```python
from build123d import *

# Parameters (mm, degrees)
SKETCH1_R          = 73.025
SKETCH1_R_2        = 42.8625
EXTRUDE1_DEPTH     = 38.1
SKETCH2_R          = 65.0875
CUT_EXTRUDE1_DEPTH = 30.1625
SKETCH3_R          = 5.55625
CUT_EXTRUDE2_DEPTH = 30.1625
CIRPATTERN1_COUNT  = 8
SKETCH5_R          = 5.55625
EXTRUDE2_DEPTH     = 7.9375
CIRPATTERN2_COUNT  = 4


with BuildPart() as part:
    # Sketch1 → Extrude1 (new body)
    with BuildSketch(Plane(origin=(0, 0, 0), x_dir=(1, 0, 0), z_dir=(0, 1, 0))):
        Circle(SKETCH1_R)
        Circle(SKETCH1_R_2, mode=Mode.SUBTRACT)
    extrude(amount=EXTRUDE1_DEPTH)

    # Sketch2 → Cut-Extrude1 (cut)
    with BuildSketch(Plane(origin=(0, 38.1, 0), x_dir=(-1, 0, 0), z_dir=(0, 1, 0))):
        Circle(SKETCH2_R)
    extrude(amount=-CUT_EXTRUDE1_DEPTH, mode=Mode.SUBTRACT)

    # Sketch3 → Cut-Extrude2 (cut)
    with BuildSketch(Plane(origin=(0, 7.9375, 0), x_dir=(-1, 0, 0), z_dir=(0, 1, 0))):
        with Locations((0, -53.975)):
            Circle(SKETCH3_R)
    cut_extrude2 = extrude(amount=-CUT_EXTRUDE2_DEPTH, mode=Mode.SUBTRACT)

    # CirPattern1: Cut-Extrude2 ×8 about axis
    cirpattern1_axis = Axis((0, 0, 0), (0, 1, 0))
    for i in range(1, CIRPATTERN1_COUNT):
        add(cut_extrude2.rotate(cirpattern1_axis, i * 360 / CIRPATTERN1_COUNT), mode=Mode.SUBTRACT)

    # Sketch5 → Extrude2 (add)
    with BuildSketch(Plane(origin=(0, 38.1, 0), x_dir=(-1, 0, 0), z_dir=(0, 1, 0))):
        with BuildLine():
            ThreePointArc((-12.413038972, -63.892872214), (0, -65.0875), (12.413038972, -63.892872214))
            Line((12.413038972, -63.892872214), (12.413038972, -53.975))
            ThreePointArc((12.413038972, -53.975), (0, -41.561961028), (-12.413038972, -53.975))
            Line((-12.413038972, -53.975), (-12.413038972, -63.892872214))
        make_face()
        with Locations((0, -53.975)):
            Circle(SKETCH5_R, mode=Mode.SUBTRACT)
    extrude2 = extrude(amount=-EXTRUDE2_DEPTH)

    # CirPattern2: Extrude2 ×4 about axis
    cirpattern2_axis = Axis((0, 0, 0), (0, 1, 0))
    for i in range(1, CIRPATTERN2_COUNT):
        add(extrude2.rotate(cirpattern2_axis, i * 360 / CIRPATTERN2_COUNT))


solid = part.part
```
Input: part model. Units: mm. Frame: model coordinates. A direction names the side the tool comes from. Round coordinates to 2 decimals unless told otherwise and drop trailing zeros. Loops run counter-clockwise (first coordinate to the right, second up) from the corner with the lowest first, then second, coordinate; pieces in that order, holes last. Notation, with made-up numbers: (80.25, 72.25) -> (120.25, 72.25) arc R17 cw to (120.25, 100.25) -> close; hole circle Ø6 at (78.25, -21.75). An arc over 180 degrees is marked (long way). Use one line per item in the form item = value. Start each with the question number.
Item 1: Mould query, pull axis Z, two halves, no side actions, for faces 4 (the face through (41.565, 34.187, -0.273)), 5 (the face through (31, 0, 31)). Classes: pulls with the +Z half, pulls with the -Z half, needs draft (parallel to the pull), parting line crosses it, or undercut.
Item 2: Section query D-D on x = 23.5. Return the cut outline in (y, z).
Item 3: Material intervals for L1, parallel to Z at x = 0, y = 36 (3 decimals); L2, parallel to Z at x = 0, y = 3.25 (1 decimal), sorted ascending. Write a range as from..to.
Item 4: Contact query for flat-ended pins moving along their axis: pin 1 Ø8.5 at (x, y) = (-61, 33.5) entering from -Z; pin 2 Ø6.5 at (y, z) = (32.5, -56.5) entering from +X; pin 3 Ø8.5 at (x, y) = (59, 35) entering from +Z; pin 4 Ø9 at (x, z) = (0, 53.975) entering from +Y. Output: stop coordinate, or through.
Item 5: Section query A-A on x = 0. Count the separate pieces of the cut face and the enclosed holes in it, then the cut area to 3 significant figures.
Item 6: Set-up query: faces 1 (the face through (-48.466, 4.024, -0.723)), 2 (the face through (-53, 30.162, -6)), 3 (the face through (12.413, 34, 59)). Return all of +Z, -Z, +X, -X, +Y, -Y with unobstructed straight access to the full face (end or side cutting, diameter ignored); none if empty.
Ans:
q1.face_4 = undercut
q1.face_5 = needs draft
q2.outline = (0, -69.14) -> (38.1, -69.14) -> (38.1, -60.7) -> (7.94, -60.7) -> (7.94, -35.85) -> (0, -35.85) -> close; (0, 35.85) -> (7.94, 35.85) -> (7.94, 60.7) -> (38.1, 60.7) -> (38.1, 69.14) -> (0, 69.14) -> close
q3.L1 = -73.025..-59.531, -48.419..-41.562, 41.562..48.419, 59.531..73.025
q3.L2 = -73..-59.5, -48.4..-42.9, 42.9..48.4, 59.5..73
q4.pin_1 = -45.96
q4.pin_2 = 49.97
q4.pin_3 = 48.32
q4.pin_4 = through
q5.separate_pieces = 6
q5.enclosed_holes = 0
q5.area = 978 mm^2
q6.face_1 = +Y, -Y
q6.face_2 = none
q6.face_3 = +Y
